Read the model definition and answer for the solid it produces. Units are mm, in the model's axes. A direction names the side the tool comes from. Give positions to 0.01 mm unless a question says otherwise; leave off trailing zeros. Loops run counter-clockwise (first coordinate to the right, second up) from the corner with the lowest first, then second, coordinate; pieces in that order, holes last.
(1) Find section A-A, the plane y = 0. State how many separate pieces and enclosed holes the cut face has, then the cut area to 3 significant figures.
(2) Determine the mould class of faces 1 (the face through (23.09, -33.287, -50.97)), 2 (the face through (1.96, 12.3, -75.56)), 3 (the face through (-48, 0, 5)), 4 (the face through (-60, 0, 5)) for opening direction X: pulls with the +X half, pulls with the -X half, needs draft (parallel to the pull), parting line crosses it, or undercut.
(3) Straight lines are drawn through the part: probe 1 along Z at (x, y) = (0, -13.95); probe 2 along Z at (x, y) = (4, -20); probe 3 along Y at (x, z) = (-45, 7.75). For each, find the intervals that lie inside material, in ascending order.
(4) Find section C-C, the plane z = -77. Write down the section's boundary in (x, y).
(5) Which of the six approach directions +Z, -Z, +X, -X, +Y, -Y give full straight-line access (tool end or side, diameter ignored) to faces 5 (the face through (12.31, 1.28, -83.25)), 6 (the face through (1.323, 10.074, -4.437)), 7 (the face through (-8.19, 12.85, -44.37))?
(6) Find section B-B, the plane x = -45. Write down the section's boundary in (y, z).
(7) Find section D-D, the plane z = -12. Write down the section's boundary in (x, y).
(8) Each of these flat-tipped pins is pushed along its axis until it touches: P1, Ø16.5, axis at x = 5, y = -3, coming from the -Z side; P2, Ø8, axis at x = -9.5, z = 2.5, coming from the -Y side; P3, Ø11, axis at x = 0, z = -79.33, coming from the +Y side; P4, Ø11, axis at y = 0, z = -79.2, coming from the -X side. Where does it stop, or does it pass through?
```python
from build123d import *

# Parameters (mm, degrees)
SKETCH1_W                = 120
SKETCH1_H                = 70
SKETCH1_R                = 3
BOSS_EXTRUDE1_DEPTH      = 10
SKETCH2_R                = 15.24
SKETCH2_R_2              = 10.16
BOSS_EXTRUDE2_DEPTH      = 90
SKETCH4_R                = 12.2
SKETCH4_R_2              = 10.2
BOSS_EXTRUDE4_DEPTH      = 27
BOSS_EXTRUDE4_DEPTH_BACK = 20
SKETCH6_R                = 4.25
CUT_EXTRUDE1_DEPTH       = 58
SKETCH7_R                = 4.25
CUT_EXTRUDE2_DEPTH       = 81
FILLET1_R                = 10
SKETCH8_R                = 10.211266942
CUT_EXTRUDE3_DEPTH       = 81


with BuildPart() as part:
    # Sketch1 → Boss-Extrude1 (new body)
    with BuildSketch(Plane.XY):
        Rectangle(SKETCH1_W, SKETCH1_H)
        with Locations((-45, 0)):
            Circle(SKETCH1_R, mode=Mode.SUBTRACT)
        with Locations((45, 0)):
            Circle(SKETCH1_R, mode=Mode.SUBTRACT)
    extrude(amount=BOSS_EXTRUDE1_DEPTH)

    # Sketch2 → Boss-Extrude2 (add)
    with BuildSketch(Plane(origin=(0, 0, 0), x_dir=(-1, 0, 0), z_dir=(0, 0, -1))):
        Circle(SKETCH2_R)
        Circle(SKETCH2_R_2, mode=Mode.SUBTRACT)
    extrude(amount=BOSS_EXTRUDE2_DEPTH)

    # Sketch4 → Boss-Extrude4 (add, two sides)
    with BuildSketch(Plane(origin=(12.998571072, -24.340292843, -4.528818833), x_dir=(0.885388994, 0.457007531, 0.085032022), z_dir=(-0.464850867, 0.870450003, 0.161958214))) as boss_extrude4_sk:
        with Locations((-4.468384796, 53.00095998)):
            Circle(SKETCH4_R)
        with Locations((-4.468384796, 53.00095998)):
            Circle(SKETCH4_R_2, mode=Mode.SUBTRACT)
    extrude(amount=BOSS_EXTRUDE4_DEPTH)
    extrude(boss_extrude4_sk.sketch, amount=-BOSS_EXTRUDE4_DEPTH_BACK)

    # Sketch6 → Cut-Extrude1 (cut)
    with BuildSketch(Plane(origin=(0, 35, 0), x_dir=(1, 0, 0), z_dir=(0, 1, 0))):
        with Locations((0, 79.330798524)):
            Circle(SKETCH6_R)
    extrude(amount=-CUT_EXTRUDE1_DEPTH, mode=Mode.SUBTRACT)

    # Sketch7 → Cut-Extrude2 (cut)
    with BuildSketch(Plane(origin=(60, 0, 0), x_dir=(0, 0, -1), z_dir=(1, 0, 0))):
        with Locations((79.196792396, 0)):
            Circle(SKETCH7_R)
    extrude(amount=-CUT_EXTRUDE2_DEPTH, mode=Mode.SUBTRACT)

    # Fillet1
    fillet1_edges = [part.edges().sort_by_distance(p)[0] for p in [
        (60, -35, 5),
        (-60, -35, 5),
        (-60, 35, 5),
        (60, 35, 5),
    ]]
    fillet(fillet1_edges, radius=FILLET1_R)

    # Sketch8 → Cut-Extrude3 (cut)
    with BuildSketch(Plane(origin=(0, 0, -90), x_dir=(-1, 0, 0), z_dir=(0, 0, -1))):
        Circle(SKETCH8_R)
    extrude(amount=-CUT_EXTRUDE3_DEPTH, mode=Mode.SUBTRACT)


solid = part.part
```
Entries:
1. separate pieces: 5
1. enclosed holes: 0
1. area: 1,900 mm2
2. face 1: pulls with the +X half
2. face 2: undercut
2. face 3: undercut
2. face 4: pulls with the -X half
3. probe 1: z = -90 to -83.58, -75.08 to 10
3. probe 2: z = -67.87 to -65.46, -48.75 to -46.35, 0 to 10
3. probe 3: y = -35 to -3, 3 to 35
4. outline: (-14.8, -3.64) arc R15.24 ccw to (-3.55, -14.82) - (-3.55, -9.57) arc R10.21 cw to (-9.54, -3.64) - close; (-14.8, 3.64) - (-9.54, 3.64) arc R10.21 cw to (-3.55, 9.57) - (-3.55, 14.82) arc R15.24 ccw to start; (3.55, -14.82) arc R15.24 ccw to (14.8, -3.64) - (9.54, -3.64) arc R10.21 cw to (3.55, -9.57) - close; (3.55, 9.57) arc R10.21 cw to (9.54, 3.64) - (14.8, 3.64) arc R15.24 ccw to (3.55, 14.82) - close
5. face 5: +X, -X
5. face 6: -Z
5. face 7: none
6. outline: (-35, 0) - (-3, 0) - (-3, 10) - (-35, 10) - close; (3, 0) - (35, 0) - (35, 10) - (3, 10) - close
7. outline: circle Ø30.48 at (0, 0); hole circle Ø20.42 at (0, 0)
8. P1: stops at z = -90
8. P2: stops at y = -35
8. P3: stops at y = 15.24
8. P4: stops at x = -15.24
